```python
from build123d import *

# Parameters (mm, degrees)
SKETCH1_R           = 1.5
BOSS_EXTRUDE1_DEPTH = 3


with BuildPart() as part:
    # Sketch1 → Boss-Extrude1 (new body)
    with BuildSketch(Plane(origin=(0, 0, 0), x_dir=(1, 0, 0), z_dir=(0, 1, 0))):
        with BuildLine():
            Line((27, 10), (-27, 10))
            Line((-27, 10), (-27, -10))
            Line((-27, -10), (21, -10))
            ThreePointArc((21, -10), (25.242640687, -8.242640687), (27, -4))
            Line((27, -4), (27, 0))
            Line((27, 0), (30, 0))
            Line((30, 0), (30, 10))
            Line((30, 10), (27, 10))
        make_face()
        with Locations(Location((24, -3.5, 0), (0, 0, 270))):
            Circle(SKETCH1_R, mode=Mode.SUBTRACT)
    extrude(amount=BOSS_EXTRUDE1_DEPTH)


solid = part.part
```
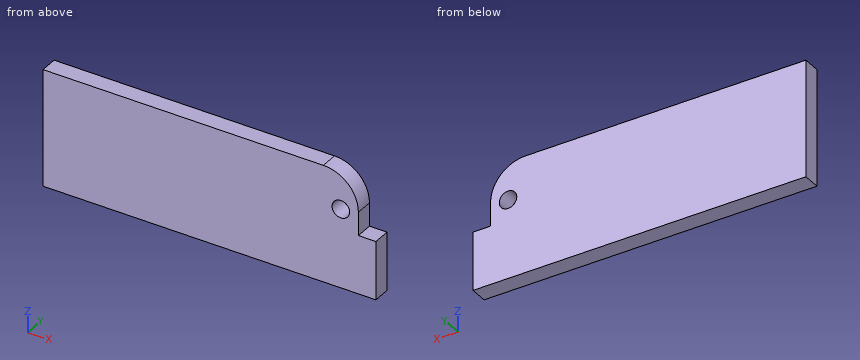
The model under review builds one solid part; all positions refer to its coordinate system, in mm. Give positions to 0.01 mm unless a question says otherwise; leave off trailing zeros. Write each loop counter-clockwise with the first axis right and the second up, starting at its lowest first coordinate (ties: lowest second). Pieces come first, ordered by that corner, then holes.
(1) Consider section D-D, the plane z = 7.5. Give the boundary of the cut face in (x, y), and give its area (3 significant figures).
(2) Consider section B-B, the plane y = 1.75. Give the boundary of the cut face in (x, z), and give its area (3 significant figures).
(3) Consider section A-A, the plane z = 3.5. Give the boundary of the cut face in (x, y), and give its area (3 significant figures).
(4) Consider section C-C, the plane x = 24. Give the boundary of the cut face in (y, z).
(5) To check wall thickness, follow L1, parallel to X at y = 1.3, z = 3.5; L2, parallel to X at y = 1.75, z = 2.5; L3, parallel to Z at x = 23, y = 2.8. State the ranges of each line that lie inside material, in increasing order.
(6) For P1, Ø0.9, axis at y = 1.5, z = 3, coming from the +X side, flat-tipped, find the tip position at first contact; note if it passes through.
Returned:
1. outline: (-27, 0) - (25.87, 0) - (25.87, 3) - (-27, 3) - close
1. area: 159 mm2
2. outline: (-27, -10) - (30, -10) - (30, 0) - (27, 0) - (27, 4) arc R6 ccw to (21, 10) - (-27, 10) - close; hole circle Ø3 at (24, 3.5)
2. area: 1,100 mm2
3. outline: (-27, 0) - (22.5, 0) - (22.5, 3) - (-27, 3) - close; (25.5, 0) - (27, 0) - (27, 3) - (25.5, 3) - close
3. area: 153 mm2
4. outline: (0, -10) - (3, -10) - (3, 2) - (0, 2) - close; (0, 5) - (3, 5) - (3, 9.2) - (0, 9.2) - close
5. L1: x = -27 to 22.5, 25.5 to 27
5. L2: x = -27 to 22.88, 25.12 to 27
5. L3: z = -10 to 2.38, 4.62 to 9.66
6. P1: stops at x = 27
